Work out the finished part from the listing and answer in its coordinate system (mm). Face numbers are marked on the shaded views. A direction names the side the tool comes from. Coordinates: 2 decimals unless noted, no trailing zeros. Loops run counter-clockwise (first coordinate to the right, second up) from the corner with the lowest first, then second, coordinate; pieces in that order, holes last.
```python
from build123d import *

# Parameters (mm, degrees)
F0_R     = 12.25
F0_W     = 8.5
F0_H     = 20
F1_DEPTH = 1.2
F2_DEPTH = 7
F3_R     = 0.5
F4_DEPTH = 5


with BuildPart() as f1:
    # F0 (on Front) → F1 (new body)
    with BuildSketch(Plane.XZ):
        Circle(F0_R)
        Rectangle(F0_W, F0_H, mode=Mode.SUBTRACT)
    extrude(amount=F1_DEPTH)

    # F0 (on Front) → F2 (join)
    with BuildSketch(Plane.XZ):
        Rectangle(F0_W, F0_H)
    extrude(amount=F2_DEPTH)

    # F3 (on face) → F4 (cut)
    with BuildSketch(Plane.XZ.offset(7)):
        with Locations((0, -7.5)):
            Circle(F3_R)
        with Locations((0, 7.5)):
            Circle(F3_R)
    extrude(amount=-F4_DEPTH, mode=Mode.SUBTRACT)


solid = f1.part
```
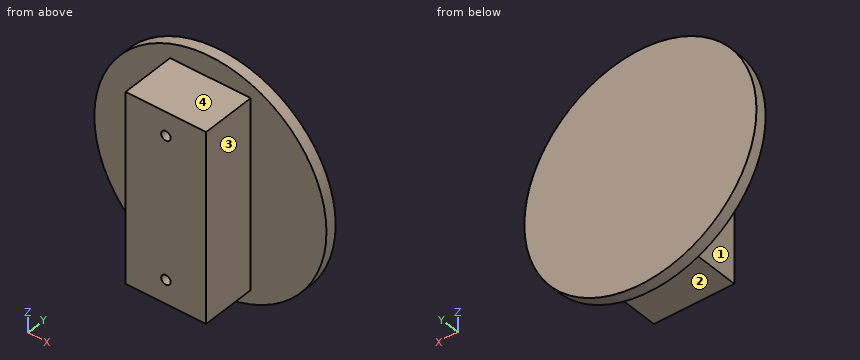
1. A cutting plane is placed at A-A, the plane y = -5. Give the vertices of the cut face in (x, z).
2. Each of these flat-tipped pins is pushed along its axis until it touches: P1, Ø1.7, axis at x = -1, y = -5, coming from the +Z side; P2, Ø0.8, axis at x = 0, z = -7.5, coming from the -Y side; P3, Ø1.5, axis at y = -3, z = 7, coming from the -X side; P4, Ø1.1, axis at x = 0, z = 7.5, coming from the -Y side. Where does it stop, or does it pass through?
3. A cutting plane is placed at B-B, the plane z = 0. Give the vertices of the cut face in (x, y), then the cut area to 3 significant figures.
4. A cutting plane is placed at C-C, the plane x = 0. Give the vertices of the cut face in (y, z).
5. A cutting plane is placed at D-D, the plane y = -1.5. Give the vertices of the cut face in (x, z), then the cut area to 3 significant figures.
6. Straight lines are drawn through the part: probe 1 along Z at (x, y) = (0, -5.2); probe 2 along X at (y, z) = (-1.75, -9.5); probe 3 along Y at (x, z) = (10.75, -1). For each, find the intervals that lie inside material, in ascending order.
7. For the marked faces 1, 2, 3 and 4, determine the directions among +Z, -Z, +X, -X, +Y, -Y from which every point of the face is accessible in a straight line to the end or side of a thin tool.
Answers below:
1. outline: (-4.25, -10) - (4.25, -10) - (4.25, 10) - (-4.25, 10) - close; hole circle Ø1 at (0, -7.5); hole circle Ø1 at (0, 7.5)
2. P1: stops at z = 10
2. P2: stops at y = -2
2. P3: stops at x = -4.25
2. P4: stops at y = -7
3. outline: (-12.25, -1.2) - (-4.25, -1.2) - (-4.25, -7) - (4.25, -7) - (4.25, -1.2) - (12.25, -1.2) - (12.25, 0) - (-12.25, 0) - close
3. area: 78.7 mm2
4. outline: (-7, -10) - (-1.2, -10) - (-1.2, -12.25) - (0, -12.25) - (0, 12.25) - (-1.2, 12.25) - (-1.2, 10) - (-7, 10) - (-7, 8) - (-2, 8) - (-2, 7) - (-7, 7) - (-7, -7) - (-2, -7) - (-2, -8) - (-7, -8) - close
5. outline: (-4.25, -10) - (4.25, -10) - (4.25, 10) - (-4.25, 10) - close
5. area: 170 mm2
6. probe 1: z = -10 to -8, -7 to 7, 8 to 10
6. probe 2: x = -4.25 to 4.25
6. probe 3: y = -1.2 to 0
7. face 1: +Z, -Z, -X, -Y
7. face 2: -Z, +X, -X, -Y
7. face 3: +Z, -Z, +X, -Y
7. face 4: +Z, +X, -X, -Y
